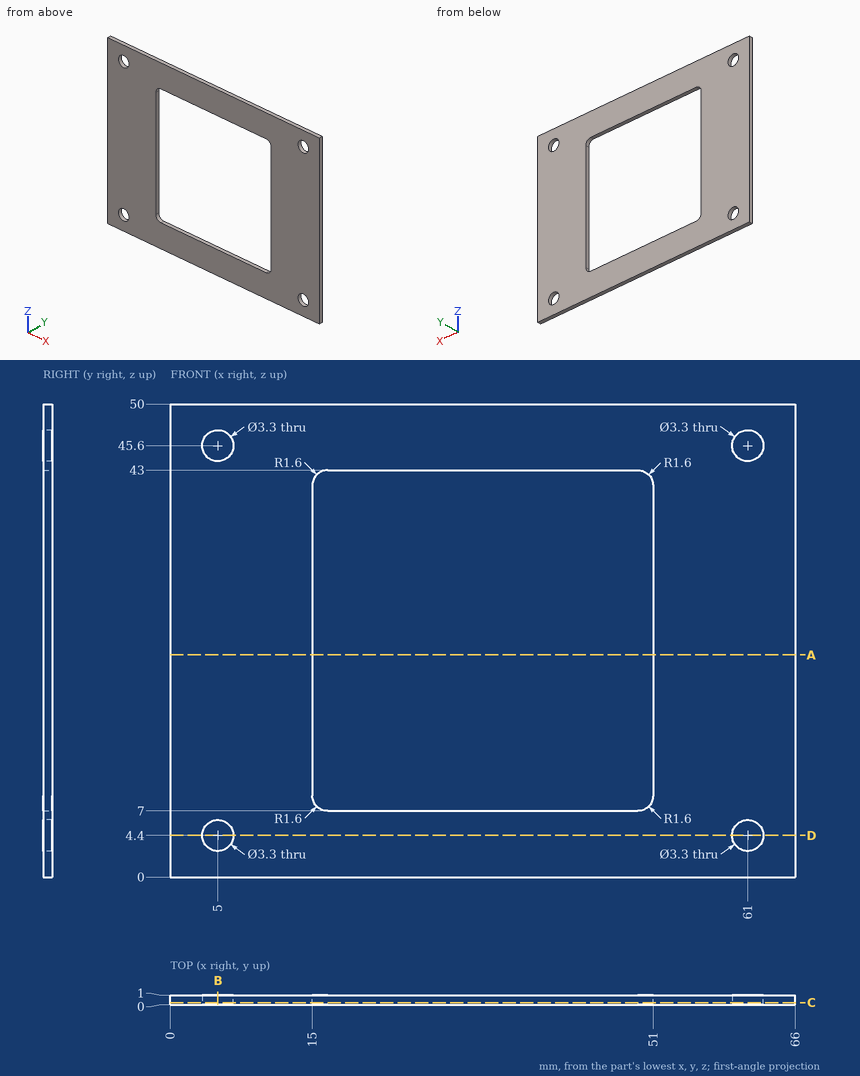
Design review of the part shown in the three views and the two pictorial views. Dimensions are in mm from the part's minimum x, y and z. Coordinates: 2 decimals unless noted, no trailing zeros. Order: outer loops, then holes, each group sorted by start corner. A loop starts at its lowest first (then second) coordinate and runs counter-clockwise, first axis right, second up.
1) Take a section at D-D, the plane z = 4.4. Give the boundary of the cut face in (x, y).
2) Clearance check with a flat-ended pin moving along its axis: pin 1 (2 mm diameter, centred on x = 61, z = 4.4, fed in from +Y). State where the tip first meets the part, or that it passes through.
3) Take a section at B-B, the plane x = 5. Give the boundary of the cut face in (y, z), and give its area (3 significant figures).
4) Wall thickness on line 1 along X through (y, z) = (0.7, 45.6); line 2 along Z through (x, y) = (61, 0.45); line 3 along Z through (x, y) = (28.5, 0.95): over which ranges is each line inside the solid? List them lowest first.
5) Take a section at A-A, the plane z = 23.5. Give the boundary of the cut face in (x, y).
6) Take a section at C-C, the plane y = 0.2. Give the boundary of the cut face in (x, z).
Returned:
1. outline: (0, 0) - (3.35, 0) - (3.35, 1) - (0, 1) - close; (6.65, 0) - (59.35, 0) - (59.35, 1) - (6.65, 1) - close; (62.65, 0) - (66, 0) - (66, 1) - (62.65, 1) - close
2. pin 1: passes through
3. outline: (0, 0) - (1, 0) - (1, 2.75) - (0, 2.75) - close; (0, 6.05) - (1, 6.05) - (1, 43.95) - (0, 43.95) - close; (0, 47.25) - (1, 47.25) - (1, 50) - (0, 50) - close
3. area: 43.4 mm2
4. line 1: x = 0 to 3.35, 6.65 to 59.35, 62.65 to 66
4. line 2: z = 0 to 2.75, 6.05 to 43.95, 47.25 to 50
4. line 3: z = 0 to 7, 43 to 50
5. outline: (0, 0) - (15, 0) - (15, 1) - (0, 1) - close; (51, 0) - (66, 0) - (66, 1) - (51, 1) - close
6. outline: (0, 0) - (66, 0) - (66, 50) - (0, 50) - close; hole circle Ø3.3 at (5, 4.4); hole circle Ø3.3 at (5, 45.6); hole (15, 8.6) arc R1.6 ccw to (16.6, 7) - (49.4, 7) arc R1.6 ccw to (51, 8.6) - (51, 41.4) arc R1.6 ccw to (49.4, 43) - (16.6, 43) arc R1.6 ccw to (15, 41.4) - close; hole circle Ø3.3 at (61, 4.4); hole circle Ø3.3 at (61, 45.6)
